Work out the finished part from the listing and answer in its coordinate system (mm). A direction names the side the tool comes from. Coordinates: 2 decimals unless noted, no trailing zeros. Loops run counter-clockwise (first coordinate to the right, second up) from the corner with the lowest first, then second, coordinate; pieces in that order, holes last. Notation, with made-up numbers: (20, 24.5) -> (58, 24.5) arc R14 ccw to (58, 36.5) -> close; hole circle Ø7 at (-20, -29). An arc over 180 degrees is marked (long way). One line per question, with ' | ' between items.
```python
from build123d import *

# Parameters (mm, degrees)
SKETCH_1_W          = 38.5
SKETCH_1_H          = 17.6
SKETCH_1_R          = 1.5
EXTRUDE_1_DEPTH     = 10
CUT_EXTRUDE_1_DEPTH = 11
SKETCH_5_W          = 38.5
SKETCH_5_H          = 17.6
SKETCH_5_R          = 1.5
EXTRUDE_6_DEPTH     = 10
SKETCH_10_W         = 31.5
SKETCH_10_H         = 17.6
EXTRUDE_7_DEPTH     = 10
CUT_EXTRUDE_5_DEPTH = 11
CUT_EXTRUDE_6_DEPTH = 11
CHAMFER_1_SIZE      = 3
CUT_EXTRUDE_8_REACH = 19.6
SKETCH_14_R         = 1.25
CUT_EXTRUDE_9_REACH = 19.6
SKETCH_15_R         = 1.25


with BuildPart() as part:
    # Sketch 1 → Extrude 1 (new body)
    with BuildSketch(Plane(origin=(0, 0, 0), x_dir=(1, 0, 0), z_dir=(0, 1, 0))):
        Rectangle(SKETCH_1_W, SKETCH_1_H)
        with Locations((-14, 5)):
            Circle(SKETCH_1_R, mode=Mode.SUBTRACT)
        with Locations((-14, -5)):
            Circle(SKETCH_1_R, mode=Mode.SUBTRACT)
        with Locations((14, -5)):
            Circle(SKETCH_1_R, mode=Mode.SUBTRACT)
        with Locations((14, 5)):
            Circle(SKETCH_1_R, mode=Mode.SUBTRACT)
    extrude(amount=EXTRUDE_1_DEPTH)

    # Sketch 2 → Cut-Extrude 1 (cut, through all)
    with BuildSketch(Plane(origin=(0, 10, 0), x_dir=(1, 0, 0), z_dir=(0, 1, 0))):
        with BuildLine():
            Line((9.7, 5.8), (-9.7, 5.8))
            ThreePointArc((-9.7, 5.8), (-10.265685425, 5.565685425), (-10.5, 5))
            ThreePointArc((-10.5, 5), (-11.525126266, 2.525126266), (-14, 1.5))
            Line((-14, 1.5), (-16.25, 1.5))
            ThreePointArc((-16.25, 1.5), (-16.957106781, 1.207106781), (-17.25, 0.5))
            Line((-17.25, 0.5), (-17.25, -0.5))
            ThreePointArc((-17.25, -0.5), (-16.957106781, -1.207106781), (-16.25, -1.5))
            Line((-16.25, -1.5), (-14, -1.5))
            ThreePointArc((-14, -1.5), (-11.525126266, -2.525126266), (-10.5, -5))
            ThreePointArc((-10.5, -5), (-10.265685425, -5.565685425), (-9.7, -5.8))
            Line((-9.7, -5.8), (9.7, -5.8))
            ThreePointArc((9.7, -5.8), (10.265685425, -5.565685425), (10.5, -5))
            ThreePointArc((10.5, -5), (11.525126266, -2.525126266), (14, -1.5))
            Line((14, -1.5), (16.25, -1.5))
            ThreePointArc((16.25, -1.5), (16.957106781, -1.207106781), (17.25, -0.5))
            Line((17.25, -0.5), (17.25, 0.5))
            ThreePointArc((17.25, 0.5), (16.957106781, 1.207106781), (16.25, 1.5))
            Line((16.25, 1.5), (14, 1.5))
            ThreePointArc((14, 1.5), (11.525126266, 2.525126266), (10.5, 5))
            ThreePointArc((10.5, 5), (10.265685425, 5.565685425), (9.7, 5.8))
        make_face()
    extrude(amount=-CUT_EXTRUDE_1_DEPTH, mode=Mode.SUBTRACT)



with BuildPart() as body_2:
    # Sketch 5 → Extrude 6 (new body)
    with BuildSketch(Plane(origin=(0, 10, 0), x_dir=(1, 0, 0), z_dir=(0, 1, 0))):
        with Locations((70, 0)):
            Rectangle(SKETCH_5_W, SKETCH_5_H)
        with Locations((56, 5)):
            Circle(SKETCH_5_R, mode=Mode.SUBTRACT)
        with Locations((84, 5)):
            Circle(SKETCH_5_R, mode=Mode.SUBTRACT)
        with Locations((84, -5)):
            Circle(SKETCH_5_R, mode=Mode.SUBTRACT)
        with Locations((56, -5)):
            Circle(SKETCH_5_R, mode=Mode.SUBTRACT)
    extrude(amount=-EXTRUDE_6_DEPTH)


with BuildPart() as part_1:
    add(part.part)

    add(body_2.part)  # Extrude 7 merges body 2
    # Sketch 10 → Extrude 7 (add)
    with BuildSketch(Plane(origin=(0, 10, 0), x_dir=(1, 0, 0), z_dir=(0, 1, 0))):
        with Locations((35, 0)):
            Rectangle(SKETCH_10_W, SKETCH_10_H)
    extrude(amount=-EXTRUDE_7_DEPTH)

    # Sketch 11 → Cut-Extrude 5 (cut, through all)
    with BuildSketch(Plane(origin=(0, 10, 0), x_dir=(1, 0, 0), z_dir=(0, 1, 0))):
        with BuildLine():
            Line((16.25, 1.5), (14, 1.5))
            ThreePointArc((14, 1.5), (11.525126266, 2.525126266), (10.5, 5))
            ThreePointArc((10.5, 5), (10.265685425, 5.565685425), (9.7, 5.8))
            Line((9.7, 5.8), (-9.7, 5.8))
            ThreePointArc((-9.7, 5.8), (-10.265685425, 5.565685425), (-10.5, 5))
            ThreePointArc((-10.5, 5), (-11.525126266, 2.525126266), (-14, 1.5))
            Line((-14, 1.5), (-16.25, 1.5))
            ThreePointArc((-16.25, 1.5), (-16.957106781, 1.207106781), (-17.25, 0.5))
            Line((-17.25, 0.5), (-17.25, -0.5))
            ThreePointArc((-17.25, -0.5), (-16.957106781, -1.207106781), (-16.25, -1.5))
            Line((-16.25, -1.5), (-14, -1.5))
            ThreePointArc((-14, -1.5), (-11.525126266, -2.525126266), (-10.5, -5))
            ThreePointArc((-10.5, -5), (-10.265685425, -5.565685425), (-9.7, -5.8))
            Line((-9.7, -5.8), (9.7, -5.8))
            ThreePointArc((9.7, -5.8), (10.265685425, -5.565685425), (10.5, -5))
            ThreePointArc((10.5, -5), (11.525126266, -2.525126266), (14, -1.5))
            Line((14, -1.5), (16.25, -1.5))
            ThreePointArc((16.25, -1.5), (16.957106781, -1.207106781), (17.25, -0.5))
            Line((17.25, -0.5), (17.25, 0.5))
            ThreePointArc((17.25, 0.5), (16.957106781, 1.207106781), (16.25, 1.5))
        make_face()
        with BuildLine():
            Line((53.75, 1.5), (56, 1.5))
            ThreePointArc((56, 1.5), (58.474873734, 2.525126266), (59.5, 5))
            ThreePointArc((59.5, 5), (59.734314575, 5.565685425), (60.3, 5.8))
            Line((60.3, 5.8), (79.7, 5.8))
            ThreePointArc((79.7, 5.8), (80.265685425, 5.565685425), (80.5, 5))
            ThreePointArc((80.5, 5), (81.525126266, 2.525126266), (84, 1.5))
            Line((84, 1.5), (86.25, 1.5))
            ThreePointArc((86.25, 1.5), (86.957106781, 1.207106781), (87.25, 0.5))
            Line((87.25, 0.5), (87.25, -0.5))
            ThreePointArc((87.25, -0.5), (86.957106781, -1.207106781), (86.25, -1.5))
            Line((86.25, -1.5), (84, -1.5))
            ThreePointArc((84, -1.5), (81.525126266, -2.525126266), (80.5, -5))
            ThreePointArc((80.5, -5), (80.265685425, -5.565685425), (79.7, -5.8))
            Line((79.7, -5.8), (60.3, -5.8))
            ThreePointArc((60.3, -5.8), (59.734314575, -5.565685425), (59.5, -5))
            ThreePointArc((59.5, -5), (58.474873734, -2.525126266), (56, -1.5))
            Line((56, -1.5), (53.75, -1.5))
            ThreePointArc((53.75, -1.5), (53.042893219, -1.207106781), (52.75, -0.5))
            Line((52.75, -0.5), (52.75, 0.5))
            ThreePointArc((52.75, 0.5), (53.042893219, 1.207106781), (53.75, 1.5))
        make_face()
    extrude(amount=-CUT_EXTRUDE_5_DEPTH, mode=Mode.SUBTRACT)

    # Sketch 12 → Cut-Extrude 6 (cut, through all)
    with BuildSketch(Plane(origin=(0, 10, 0), x_dir=(1, 0, 0), z_dir=(0, 1, 0))):
        with BuildLine():
            Line((22.5, 6), (47.5, 6))
            ThreePointArc((47.5, 6), (49.5, 4), (47.5, 2))
            Line((47.5, 2), (22.5, 2))
            ThreePointArc((22.5, 2), (20.5, 4), (22.5, 6))
        make_face()
        with BuildLine():
            Line((22.5, -6), (47.5, -6))
            ThreePointArc((47.5, -6), (49.5, -4), (47.5, -2))
            Line((47.5, -2), (22.5, -2))
            ThreePointArc((22.5, -2), (20.5, -4), (22.5, -6))
        make_face()
    extrude(amount=-CUT_EXTRUDE_6_DEPTH, mode=Mode.SUBTRACT)

    # Chamfer 1
    chamfer_1_edges = [part_1.edges().sort_by_distance(p)[0] for p in [
        (89.25, 5, 8.8),
        (89.25, 5, -8.8),
        (-19.25, 5, 8.8),
        (-19.25, 5, -8.8),
    ]]
    chamfer(chamfer_1_edges, length=CHAMFER_1_SIZE)

    # Sketch 14 → Cut-Extrude 8 (cut, up to next)
    with BuildSketch(Plane(origin=(0, 0, -8.8), x_dir=(-1, 0, 0), z_dir=(0, 0, -1)), mode=Mode.PRIVATE) as cut_extrude_8_sk1:
        with Locations((-47, 5)):
            Circle(SKETCH_14_R)
    cut_extrude_8_tool1 = extrude(cut_extrude_8_sk1.sketch, amount=-CUT_EXTRUDE_8_REACH, mode=Mode.PRIVATE) & part_1.part
    add(cut_extrude_8_tool1.solids().sort_by_distance((47, 5, -8.8))[0], mode=Mode.SUBTRACT)
    # Sketch 14 → Cut-Extrude 8 (cut, up to next)
    with BuildSketch(Plane(origin=(0, 0, -8.8), x_dir=(-1, 0, 0), z_dir=(0, 0, -1)), mode=Mode.PRIVATE) as cut_extrude_8_sk2:
        with Locations((-78.5, 5)):
            Circle(SKETCH_14_R)
    cut_extrude_8_tool2 = extrude(cut_extrude_8_sk2.sketch, amount=-CUT_EXTRUDE_8_REACH, mode=Mode.PRIVATE) & part_1.part
    add(cut_extrude_8_tool2.solids().sort_by_distance((78.5, 5, -8.8))[0], mode=Mode.SUBTRACT)
    # Sketch 14 → Cut-Extrude 8 (cut, up to next)
    with BuildSketch(Plane(origin=(0, 0, -8.8), x_dir=(-1, 0, 0), z_dir=(0, 0, -1)), mode=Mode.PRIVATE) as cut_extrude_8_sk3:
        with Locations((-61.5, 5)):
            Circle(SKETCH_14_R)
    cut_extrude_8_tool3 = extrude(cut_extrude_8_sk3.sketch, amount=-CUT_EXTRUDE_8_REACH, mode=Mode.PRIVATE) & part_1.part
    add(cut_extrude_8_tool3.solids().sort_by_distance((61.5, 5, -8.8))[0], mode=Mode.SUBTRACT)
    # Sketch 14 → Cut-Extrude 8 (cut, up to next)
    with BuildSketch(Plane(origin=(0, 0, -8.8), x_dir=(-1, 0, 0), z_dir=(0, 0, -1)), mode=Mode.PRIVATE) as cut_extrude_8_sk4:
        with Locations((-23, 5)):
            Circle(SKETCH_14_R)
    cut_extrude_8_tool4 = extrude(cut_extrude_8_sk4.sketch, amount=-CUT_EXTRUDE_8_REACH, mode=Mode.PRIVATE) & part_1.part
    add(cut_extrude_8_tool4.solids().sort_by_distance((23, 5, -8.8))[0], mode=Mode.SUBTRACT)
    # Sketch 14 → Cut-Extrude 8 (cut, up to next)
    with BuildSketch(Plane(origin=(0, 0, -8.8), x_dir=(-1, 0, 0), z_dir=(0, 0, -1)), mode=Mode.PRIVATE) as cut_extrude_8_sk5:
        with Locations((-8.5, 5)):
            Circle(SKETCH_14_R)
    cut_extrude_8_tool5 = extrude(cut_extrude_8_sk5.sketch, amount=-CUT_EXTRUDE_8_REACH, mode=Mode.PRIVATE) & part_1.part
    add(cut_extrude_8_tool5.solids().sort_by_distance((8.5, 5, -8.8))[0], mode=Mode.SUBTRACT)
    # Sketch 14 → Cut-Extrude 8 (cut, up to next)
    with BuildSketch(Plane(origin=(0, 0, -8.8), x_dir=(-1, 0, 0), z_dir=(0, 0, -1)), mode=Mode.PRIVATE) as cut_extrude_8_sk6:
        with Locations((8.5, 5)):
            Circle(SKETCH_14_R)
    cut_extrude_8_tool6 = extrude(cut_extrude_8_sk6.sketch, amount=-CUT_EXTRUDE_8_REACH, mode=Mode.PRIVATE) & part_1.part
    add(cut_extrude_8_tool6.solids().sort_by_distance((-8.5, 5, -8.8))[0], mode=Mode.SUBTRACT)

    # Sketch 15 → Cut-Extrude 9 (cut, up to next)
    with BuildSketch(Plane.XY.offset(8.8), mode=Mode.PRIVATE) as cut_extrude_9_sk1:
        with Locations((-8.5, 5)):
            Circle(SKETCH_15_R)
    cut_extrude_9_tool1 = extrude(cut_extrude_9_sk1.sketch, amount=-CUT_EXTRUDE_9_REACH, mode=Mode.PRIVATE) & part_1.part
    add(cut_extrude_9_tool1.solids().sort_by_distance((-8.5, 5, 8.8))[0], mode=Mode.SUBTRACT)
    # Sketch 15 → Cut-Extrude 9 (cut, up to next)
    with BuildSketch(Plane.XY.offset(8.8), mode=Mode.PRIVATE) as cut_extrude_9_sk2:
        with Locations((8.5, 5)):
            Circle(SKETCH_15_R)
    cut_extrude_9_tool2 = extrude(cut_extrude_9_sk2.sketch, amount=-CUT_EXTRUDE_9_REACH, mode=Mode.PRIVATE) & part_1.part
    add(cut_extrude_9_tool2.solids().sort_by_distance((8.5, 5, 8.8))[0], mode=Mode.SUBTRACT)
    # Sketch 15 → Cut-Extrude 9 (cut, up to next)
    with BuildSketch(Plane.XY.offset(8.8), mode=Mode.PRIVATE) as cut_extrude_9_sk3:
        with Locations((23, 5)):
            Circle(SKETCH_15_R)
    cut_extrude_9_tool3 = extrude(cut_extrude_9_sk3.sketch, amount=-CUT_EXTRUDE_9_REACH, mode=Mode.PRIVATE) & part_1.part
    add(cut_extrude_9_tool3.solids().sort_by_distance((23, 5, 8.8))[0], mode=Mode.SUBTRACT)
    # Sketch 15 → Cut-Extrude 9 (cut, up to next)
    with BuildSketch(Plane.XY.offset(8.8), mode=Mode.PRIVATE) as cut_extrude_9_sk4:
        with Locations((47, 5)):
            Circle(SKETCH_15_R)
    cut_extrude_9_tool4 = extrude(cut_extrude_9_sk4.sketch, amount=-CUT_EXTRUDE_9_REACH, mode=Mode.PRIVATE) & part_1.part
    add(cut_extrude_9_tool4.solids().sort_by_distance((47, 5, 8.8))[0], mode=Mode.SUBTRACT)
    # Sketch 15 → Cut-Extrude 9 (cut, up to next)
    with BuildSketch(Plane.XY.offset(8.8), mode=Mode.PRIVATE) as cut_extrude_9_sk5:
        with Locations((61.5, 5)):
            Circle(SKETCH_15_R)
    cut_extrude_9_tool5 = extrude(cut_extrude_9_sk5.sketch, amount=-CUT_EXTRUDE_9_REACH, mode=Mode.PRIVATE) & part_1.part
    add(cut_extrude_9_tool5.solids().sort_by_distance((61.5, 5, 8.8))[0], mode=Mode.SUBTRACT)
    # Sketch 15 → Cut-Extrude 9 (cut, up to next)
    with BuildSketch(Plane.XY.offset(8.8), mode=Mode.PRIVATE) as cut_extrude_9_sk6:
        with Locations((78.5, 5)):
            Circle(SKETCH_15_R)
    cut_extrude_9_tool6 = extrude(cut_extrude_9_sk6.sketch, amount=-CUT_EXTRUDE_9_REACH, mode=Mode.PRIVATE) & part_1.part
    add(cut_extrude_9_tool6.solids().sort_by_distance((78.5, 5, 8.8))[0], mode=Mode.SUBTRACT)


solid = part_1.part
```
1) The mould has two halves that part along Z. Classify faces 4 (the face through (-15.5, 4.93, 4.93)), 5 (the face through (34, 10, 0)), 6 (the face through (-17.73, 4.93, -7.32)): released by +Z, released by -Z, zero draft, split by the parting line, or undercut.
Check values:
face 4: undercut | face 5: zero draft | face 6: released by -Z
2) For faces 1 (the face through (34, 0, 0)), 2 (the face through (47.99, 4.24, -7.35)), 3 (the face through (81.5, 5.07, -2.55)), determine the directions among +Z, -Z, +X, -X, +Y, -Y from which every point of the face is accessible in a straight line to the end or side of a thin tool.
Check values:
face 1: +Z, -Z, +X, -X, -Y | face 2: -Z | face 3: +Y, -Y
3) Find section B-B (z = -7.5). Write down the section's boundary in (x, y), plus the area to 3 significant figures.
Check values:
outline: (-17.55, 0) -> (87.55, 0) -> (87.55, 10) -> (-17.55, 10) -> close; hole circle Ø2.5 at (-8.5, 5); hole circle Ø2.5 at (8.5, 5); hole circle Ø2.5 at (23, 5); hole circle Ø2.5 at (47, 5); hole circle Ø2.5 at (61.5, 5); hole circle Ø2.5 at (78.5, 5) | area: 1,020 mm^2
4) Find section C-C (y = 7.5). State how many separate pieces and enclosed holes the cut face has, plus the area to 3 significant figures.
Check values:
separate pieces: 1 | enclosed holes: 12 | area: 1,020 mm^2
5) A flat-ended cylindrical pin translates along its axis: pin 1 (2 mm diameter, centred on x = -8.5, y = 5, fed in from +Z). Find the tip coordinate at first contact, or state that the pin passes through.
Check values:
pin 1: passes through
6) Find the intervals of material crossed by line 1 along Z through (x, y) = (41, 2); line 2 along Z through (x, y) = (84, 4); line 3 along Z through (x, y) = (74, 2.25), in increasing order.
Check values:
line 1: z = -8.8 to -6, -2 to 2, 6 to 8.8 | line 2: z = -8.8 to -6.5, -3.5 to -1.5, 1.5 to 3.5, 6.5 to 8.8 | line 3: z = -8.8 to -5.8, 5.8 to 8.8
7) Find section A-A (x = 78.5). Write down the section's boundary in (y, z).
Check values:
outline: (0, -8.8) -> (3.75, -8.8) -> (3.75, -5.8) -> (0, -5.8) -> close; (0, 5.8) -> (3.75, 5.8) -> (3.75, 8.8) -> (0, 8.8) -> close; (6.25, -8.8) -> (10, -8.8) -> (10, -5.8) -> (6.25, -5.8) -> close; (6.25, 5.8) -> (10, 5.8) -> (10, 8.8) -> (6.25, 8.8) -> close
